The drawing under review shows one solid part. Ordinate dimensions are in mm from its lowest x, y, z. A direction names the side the tool comes from. Give positions to 0.01 mm unless a question says otherwise; leave off trailing zeros. Order: outer loops, then holes, each group sorted by start corner. A loop starts at its lowest first (then second) coordinate and runs counter-clockwise, first axis right, second up. Notation, with made-up numbers: (-3, 70.5) - (2, 70.5) arc R16 ccw to (2, 97.5) - close; hole circle Ø11 at (71.5, 59). An arc over 180 degrees is marked (long way). Use CSV: the item, a comma, the result in double quotes. Start each with the question number.
1. To check wall thickness, follow line 1 (Z direction, x = 15.75, y = 6.5); line 2 (X direction, y = 10.5, z = 2.55) (1 decimal); line 3 (Y direction, x = 13, z = 0.6). State the ranges of each line that lie inside material, in increasing order. Write a range as [from, to].
2. Take a section at A-A, the plane z = 2.65. State the section outline as (x, y) points.
3. Take a section at D-D, the plane z = 0.5. State the section outline as (x, y) points.
4. For pin 1 (2 mm diameter, centred on y = 5, z = 3, fed in from +X) (1 decimal); pin 2 (3.5 mm diameter, centred on x = 11.5, y = 8, fed in from +Z); pin 3 (1.5 mm diameter, centred on y = 8, z = 1.5, fed in from -X); pin 4 (0.8 mm diameter, centred on y = 8, z = 0.5, fed in from -X) (1 decimal), all flat-tipped, find the tip position at first contact; note any pin that passes through.
5. Take a section at C-C, the plane y = 8.75. State the section outline as (x, z) points.
6. Machinability: for the marked faces 5, 6 and 7, which of the approach directions +Z, -Z, +X, -X, +Y, -Y give a long, thin tool a straight path to every point of the face, cutting with its end or side? Answer none if there is none.
7. Draft analysis for pull direction X (two halves, no side actions). For the marked faces 1, 2, 3 and 4, state which applies: released by +X, released by -X, zero draft, split by the parting line, or undercut.
8. Take a section at B-B, the plane x = 6.5. State the section outline as (y, z) points.
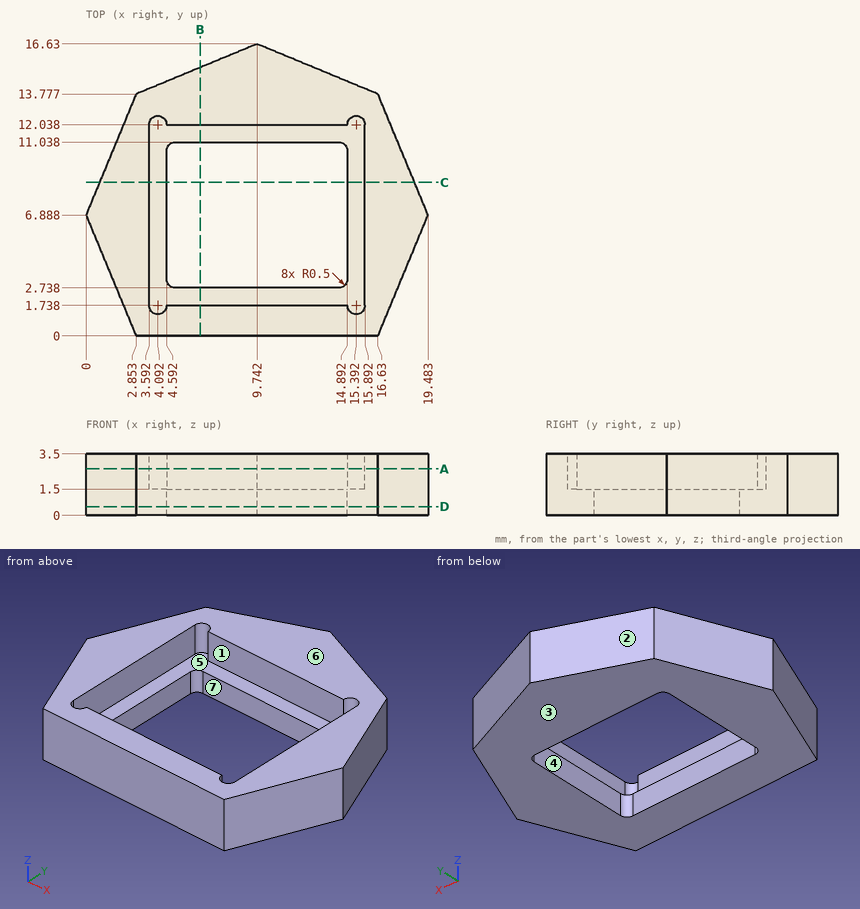
Determined:
1,line 1,"z = [0, 1.5]"
1,line 2,"x = [1.5, 3.6], [15.9, 18]"
1,line 3,"y = [0, 2.74], [11.04, 15.28]"
2,outline,"(0, 6.89) - (2.85, 0) - (16.63, 0) - (19.48, 6.89) - (16.63, 13.78) - (9.74, 16.63) - (2.85, 13.78) - close; hole (3.59, 1.74) arc R0.5 ccw to (4.59, 1.74) - (14.89, 1.74) arc R0.5 ccw to (15.89, 1.74) - (15.89, 12.04) arc R0.5 ccw to (14.89, 12.04) - (4.59, 12.04) arc R0.5 ccw to (3.59, 12.04) - close"
3,outline,"(0, 6.89) - (2.85, 0) - (16.63, 0) - (19.48, 6.89) - (16.63, 13.78) - (9.74, 16.63) - (2.85, 13.78) - close; hole (4.59, 3.24) arc R0.5 ccw to (5.09, 2.74) - (14.39, 2.74) arc R0.5 ccw to (14.89, 3.24) - (14.89, 10.54) arc R0.5 ccw to (14.39, 11.04) - (5.09, 11.04) arc R0.5 ccw to (4.59, 10.54) - close"
4,pin 1,"stops at x = 19.1"
4,pin 2,"passes through"
4,pin 3,"stops at x = 0.15"
4,pin 4,"stops at x = 0.3"
5,outline,"(0.77, 0) - (4.59, 0) - (4.59, 1.5) - (3.59, 1.5) - (3.59, 3.5) - (0.77, 3.5) - close; (14.89, 0) - (18.71, 0) - (18.71, 3.5) - (15.89, 3.5) - (15.89, 1.5) - (14.89, 1.5) - close"
6,face 5,"+Z"
6,face 6,"+Z, +X, -X, +Y, -Y"
6,face 7,"+Z, -Z"
7,face 1,"undercut"
7,face 2,"released by -X"
7,face 3,"zero draft"
7,face 4,"undercut"
8,outline,"(0, 0) - (2.74, 0) - (2.74, 1.5) - (1.74, 1.5) - (1.74, 3.5) - (0, 3.5) - close; (11.04, 0) - (15.29, 0) - (15.29, 3.5) - (12.04, 3.5) - (12.04, 1.5) - (11.04, 1.5) - close"
